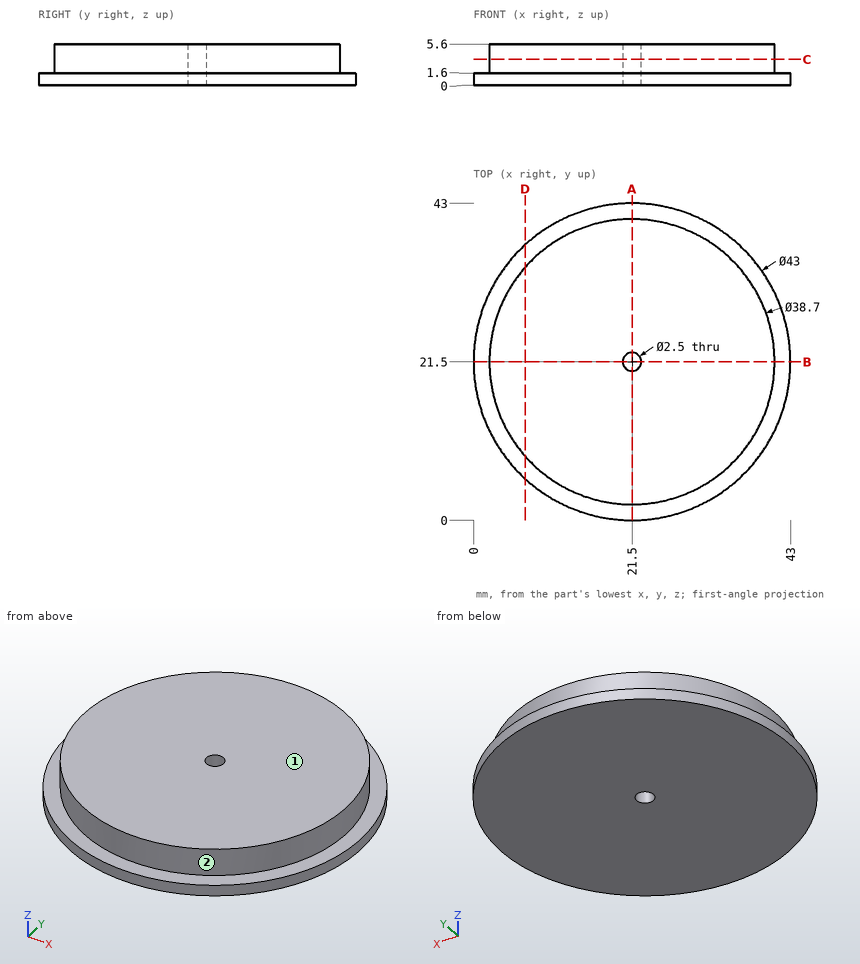
Geometry: see drawing. Coordinates: mm, zero at the bounding-box minimum. A direction names the side the tool comes from. Round coordinates to 2 decimals unless told otherwise and drop trailing zeros. Write each loop counter-clockwise with the first axis right and the second up, starting at its lowest first coordinate (ties: lowest second). Pieces come first, ordered by that corner, then holes. Notation, with made-up numbers: M 85.25,5.5 L 90.25,5.5 A12 ccw 90.25,28.5 Z; hole C 1.25,73 d4. An arc over 180 degrees is marked long. Answer in a Markdown table with one row per item. Add a question column.
(1) Reachability of the marked faces 1 and 2 from +Z, -Z, +X, -X, +Y, -Y: full face, straight path, thin tool, end or side. Return the list, or none.
(2) Contact query for flat-ended pins moving along their axis: pin 1 (1 mm diameter, centred on x = 21.5, z = 1.5, fed in from +Y); pin 2 (1 mm diameter, centred on y = 11, z = 3, fed in from +X); pin 3 (2 mm diameter, centred on y = 6, z = 1, fed in from +X). Output: stop coordinate, or through.
(3) Cut plane D-D, the plane x = 7. Return the cut outline in (y, z).
(4) Cut plane A-A, the plane x = 21.5. Return the cut outline in (y, z), then the cut area to 3 significant figures.
(5) Cut plane C-C, the plane z = 3.5. Return the cut outline in (x, y).
(6) Ray query, L1, parallel to Y at x = 21.5, z = 1.4; L2, parallel to Y at x = 21.5, z = 3.35; L3, parallel to Z at x = 14, y = 39.5. Return the intervals inside material, ascending.
Established:
| question | item | result |
|---|---|---|
| 1 | face 1 | +Z, +X, -X, +Y, -Y |
| 1 | face 2 | +Z |
| 2 | pin 1 | y = 43 |
| 2 | pin 2 | x = 38.07 |
| 2 | pin 3 | x = 37.37 |
| 3 | outline | M 5.63,0 L 37.37,0 L 37.37,1.6 L 34.31,1.6 L 34.31,5.6 L 8.69,5.6 L 8.69,1.6 L 5.63,1.6 Z |
| 4 | outline | M 0,0 L 20.25,0 L 20.25,5.6 L 2.15,5.6 L 2.15,1.6 L 0,1.6 Z; M 22.75,0 L 43,0 L 43,1.6 L 40.85,1.6 L 40.85,5.6 L 22.75,5.6 Z |
| 4 | area | 210 mm² |
| 5 | outline | C 21.5,21.5 d38.7; hole C 21.5,21.5 d2.5 |
| 6 | L1 | 0 to 20.25, 22.75 to 43 |
| 6 | L2 | 2.15 to 20.25, 22.75 to 40.85 |
| 6 | L3 | 0 to 1.6 |
